Model file for the job. Use its own axes, mm. Round coordinates to 2 decimals unless told otherwise and drop trailing zeros. Loops run counter-clockwise (first coordinate to the right, second up) from the corner with the lowest first, then second, coordinate; pieces in that order, holes last. Notation, with made-up numbers: (-36, 51) -> (-22, 51) arc R15 ccw to (-22, 64) -> close; hole circle Ø9 at (-9.75, 1.5). An arc over 180 degrees is marked (long way). Use a Markdown table: item, result.
from build123d import *

# Parameters (mm, degrees)
F1_DEPTH       = 25.4
F2_D           = 8.7376
F2_DEPTH       = 29.6333418
F2_CSINK_D     = 16.6624
F2_CSINK_ANGLE = 82
F2_TIP         = 2.6250398724
F4_D           = 19.05


# Not quite as in the source:
# - a feature names something its author has since deleted; it is built from what else it names


with BuildPart() as f1:
    # F0 (on Top) → F1 (new body)
    with BuildSketch(Plane.XY):
        Polygon((36.5125, -15.875), (36.5125, 15.875), (0, 15.875), (-36.5125, 15.875), (-36.5125, -15.875), align=None)
    extrude(amount=-F1_DEPTH)

    # F2
    with Locations(Plane.XY):
        with Locations((-23.01875, 0), (23.01875, 0)):
            CounterSinkHole(F2_D / 2, F2_CSINK_D / 2, depth=F2_DEPTH, counter_sink_angle=F2_CSINK_ANGLE)
            with Locations((0, 0, -(F2_DEPTH + F2_TIP / 2))):  # 118° drill point
                Cone(0, F2_D / 2, F2_TIP, mode=Mode.SUBTRACT)

    # F4 (through all)
    with Locations(Plane.XZ.offset(15.875)):
        with Locations((0, -25.4)):
            Hole(F4_D / 2)


solid = f1.part
Q1. Band-saw the part on A-A, the plane y = 0. Give the number of separate pieces and of enclosed holes in the cut face, plus the area to 3 significant figures.
Results list:
| item | result |
|---|---|
| separate pieces | 3 |
| enclosed holes | 0 |
| area | 1,230 mm² |
Q2. Band-saw the part on D-D, the plane x = 0. Give the cut face in (y, z) (3 decimals).
Results list:
| item | result |
|---|---|
| outline | (-15.875, -15.875) -> (15.875, -15.875) -> (15.875, 0) -> (-15.875, 0) -> close |
Q3. Drill centre lines: L1, parallel to X at y = 0, z = -13; L2, parallel to X at y = 5, z = -3; L3, parallel to X at y = -0.5, z = -20. Where is each one in solid material? Low to high. Write a range as from..to.
Results list:
| item | result |
|---|---|
| L1 | x = -36.51..-27.39, -18.65..18.65, 27.39..36.51 |
| L2 | x = -36.51..-25.8, -20.23..20.23, 25.8..36.51 |
| L3 | x = -36.51..-27.36, -18.68..-7.85, 7.85..18.68, 27.36..36.51 |
Q4. Pull direction Y, two halves, no side cores. Call faces 1 (the face through (27.576, 0.201, -4.337)), 2 (the face through (1, 15.875, -13)), 3 (the face through (-36.512, 0, -13)): released by +Y, released by -Y, zero draft, split by the parting line, or undercut.
Results list:
| item | result |
|---|---|
| face 1 | undercut |
| face 2 | released by +Y |
| face 3 | zero draft |
Q5. Band-saw the part on B-B, the plane z = -22. Give the cut face in (x, y) (1 decimal).
Results list:
| item | result |
|---|---|
| outline | (-36.5, -15.9) -> (-8.9, -15.9) -> (-8.9, 15.9) -> (-36.5, 15.9) -> close; (8.9, -15.9) -> (36.5, -15.9) -> (36.5, 15.9) -> (8.9, 15.9) -> close; hole circle Ø8.7 at (-23, 0); hole circle Ø8.7 at (23, 0) |
